Can you work these out from the drawing? Everything is in mm from the part's minimum corner. Give positions to 0.01 mm unless a question says otherwise; leave off trailing zeros. Write each loop counter-clockwise with the first axis right and the second up, starting at its lowest first coordinate (ties: lowest second). Pieces come first, ordered by that corner, then holes. Notation, with made-up numbers: (-15, -36) -> (41, -36) arc R6 cw to (41, -26) -> close; hole circle Ø2 at (12, 21.5). An arc over 180 degrees is marked (long way). Return JSON: item names as keys, results as strings.
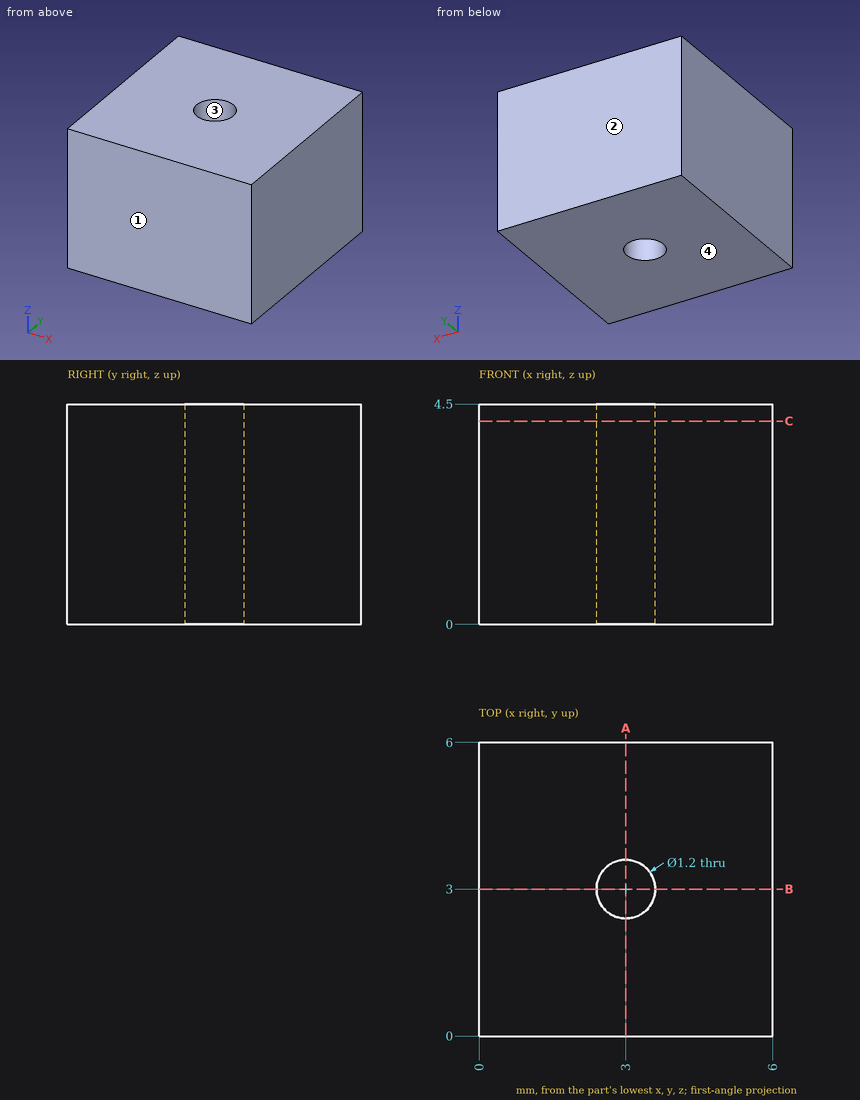
1. If I drill on line 1 (X direction, y = 3, z = 2.7); line 2 (X direction, y = 3.3, z = 3), over which ranges is the centre line in solid material (lowest first)? Write a range as [from, to].
Taken from the geometry:
{"line 1": "x = [0, 2.4], [3.6, 6]", "line 2": "x = [0, 2.48], [3.52, 6]"}
2. If we mould it in two halves opening along Y, with no side actions, what happens to the marked faces 1, 2, 3 and 4? For each: released by +Y, released by -Y, zero draft, split by the parting line, or undercut.
Taken from the geometry:
{"face 1": "released by -Y", "face 2": "released by +Y", "face 3": "undercut", "face 4": "zero draft"}
3. Suppose I cut it at A-A, the plane x = 3. List the corners of the cut face in (y, z) for me, and give its area (3 significant figures).
Taken from the geometry:
{"outline": "(0, 0) -> (2.4, 0) -> (2.4, 4.5) -> (0, 4.5) -> close; (3.6, 0) -> (6, 0) -> (6, 4.5) -> (3.6, 4.5) -> close", "area": "21.6 mm²"}
4. Suppose I cut it at C-C, the plane z = 4.15. List the corners of the cut face in (x, y) for me.
Taken from the geometry:
{"outline": "(0, 0) -> (6, 0) -> (6, 6) -> (0, 6) -> close; hole circle Ø1.2 at (3, 3)"}
